Autodesk Inventor part; units mm, degrees
ref_plane "YZ Plane" through (0, 0, 0) normal (1, 0, 0) x (0, 1, 0)
ref_plane "XZ Plane" through (0, 0, 0) normal (0, 1, 0) x (-1, 0, 0)
ref_plane "XY Plane" through (0, 0, 0) normal (0, 0, 1) x (1, 0, 0)
sketch "Sketch1" plane through (0, 0, 0) normal (0, 0, 1) x (1, 0, 0)
  circle A0 centre (4, 4) radius 1.2
  circle A1 centre (4, 4) radius 1.5
  point P0 (0, 0)
  dimension "d0" = 3
extrude "Extrusion1" add sketch "Sketch1" against normal blind 6 contours A0 | A1
sketch "Sketch2" plane through (4, 4, 0) normal (0, 0, 1) x (1, 0, 0)
  circle A0 centre (0, 0) radius 1.5
  circle A1 centre (0, 0) radius 2.8
  point P0 (-4, -4)
  dimension "d3" = 5.6
extrude "Extrusion2" add sketch "Sketch2" along normal blind 3 contours A0 | A1
fillet "Fillet1" radius 0.3 1 edges at (1.2, 4, 3)
sketch "Sketch3" plane through (4, 4, 0) normal (0, 0, -1) x (-1, 0, 0)
  circle A0 centre (0, 0) radius 2.8
  circle A1 centre (0, 0) radius 1.5
  circle A2 centre (0, 0) radius 2.75
  point P0 (4, -4)
  dimension "d7" = 5.5
extrude "Extrusion3" cut sketch "Sketch3" against normal blind 0.5 contours A0
sketch "Sketch4" plane through (4, 4, 3) normal (0, 0, 1) x (1, 0, 0)
  circle A0 centre (0, 0) radius 2.5
  line L0 (0.7217, 1.25) -> (1.4434, 0)
  line L1 (1.4434, 0) -> (0.7217, -1.25)
  line L2 (0.7217, -1.25) -> (-0.7217, -1.25)
  line L3 (-0.7217, -1.25) -> (-1.4434, 0)
  line L4 (-1.4434, 0) -> (-0.7217, 1.25)
  line L5 (-0.7217, 1.25) -> (0.7217, 1.25)
  point P0 (-4, -4)
  dimension "d10" = 2.5
extrude "Extrusion4" cut sketch "Sketch4" against normal blind 2 contours L0 L1 L2 L3 L4 L5
thread "Thread1"
properties part number "m3 6" material "Steel"
Source: CAD feature listing. Evaluate the final solid. Frame: model axes, mm. A direction names the side the tool comes from. Round coordinates to 2 decimals unless told otherwise and drop trailing zeros. Loops run counter-clockwise (first coordinate to the right, second up) from the corner with the lowest first, then second, coordinate; pieces in that order, holes last.
Q1. Ray query, line 1 (Y direction, x = 5.1, z = 2); line 2 (Z direction, x = 6, y = 3.6); line 3 (Y direction, x = 4.8, z = 2.5). Return the intervals inside material, ascending.
Q2. Section B-B, the plane z = -0.75. Return loops of the section in (x, y).
Q3. Section A-A, the plane x = 4. Return loops of the section in (y, z), plus the area to 3 significant figures.
Q4. First-contact query: P1, Ø0.7, axis at x = 4.5, z = 2, coming from the -Y side; P2, Ø1.5, axis at x = 6, z = -4.5, coming from the -Y side; P3, Ø0.8, axis at x = 4, y = 4, coming from the +Z side. Flat tips, straight axial feed; report the tip coordinate or a pass-through.
Q5. Mould query, pull axis Y, two halves, no side actions, for faces 4 (the face through (2.73, 1.56, 0.25)), 5 (the face through (4, 4, 1)), 6 (the face through (4, 4, -6)). Classes: pulls with the +Y half, pulls with the -Y half, needs draft (parallel to the pull), parting line crosses it, or undercut.
Q6. Access query for faces 1 (the face through (5.2, 2.8, 0)), 2 (the face through (5.1, 2.9, 3)), 3 (the face through (2.912, 4.616, 2.014)). Directions: +Z, -Z, +X, -X, +Y, -Y. A direction counts if a zero-diameter tool reaches every point of the face in a straight line with its end or side. Return the directions, or none.
Solutions:
1. line 1: y = 1.43 to 3.41, 4.59 to 6.57
1. line 2: z = 0 to 3
1. line 3: y = 1.32 to 2.89, 5.11 to 6.68
2. outline: circle Ø3 at (4, 4)
3. outline: (1.2, 0.5) - (1.25, 0.5) - (1.25, 0) - (2.5, 0) - (2.5, -6) - (5.5, -6) - (5.5, 0) - (6.75, 0) - (6.75, 0.5) - (6.8, 0.5) - (6.8, 2.7) arc R0.3 ccw to (6.5, 3) - (5.25, 3) - (5.25, 1) - (2.75, 1) - (2.75, 3) - (1.5, 3) arc R0.3 ccw to (1.2, 2.7) - close
3. area: 29.7 mm2
4. P1: stops at y = 1.2
4. P2: stops at y = 3.17
4. P3: stops at z = 1
5. face 4: parting line crosses it
5. face 5: undercut
5. face 6: needs draft
6. face 1: -Z
6. face 2: +Z, +X, -X, +Y, -Y
6. face 3: +Z
